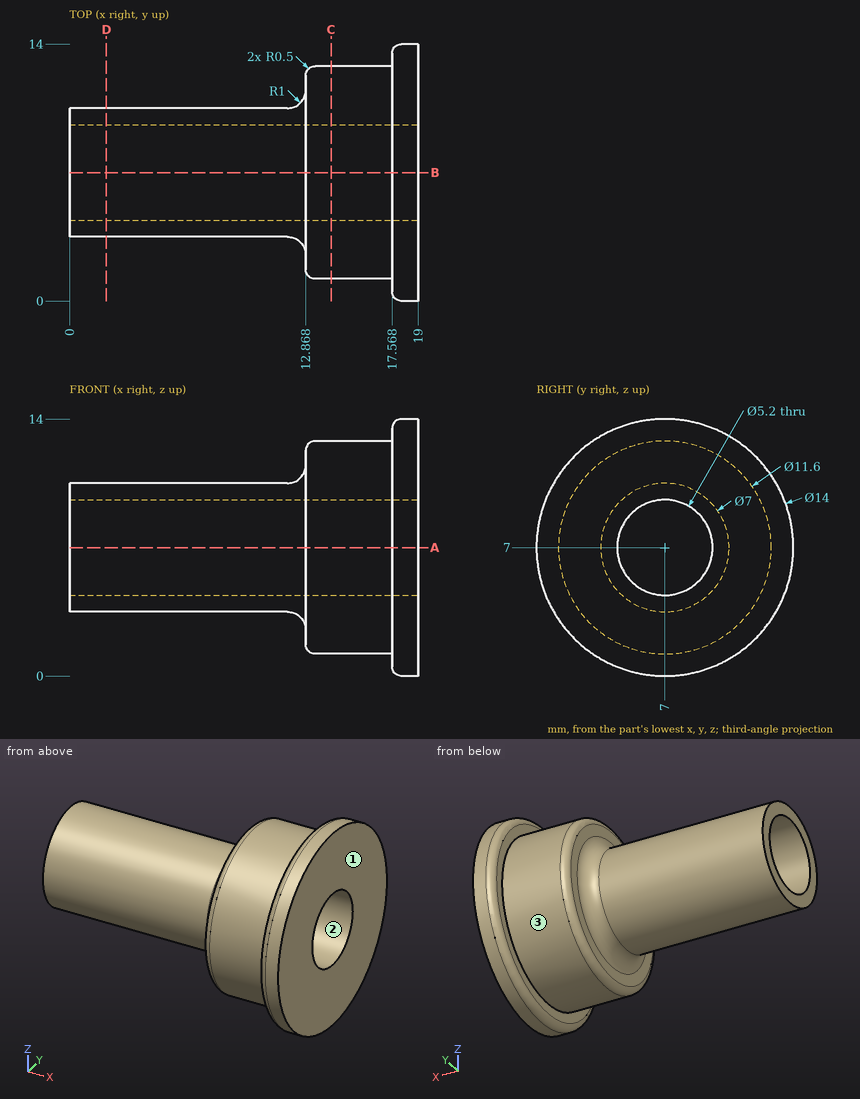
Drawing for the job (mm, zero at the part's lowest x, y, z). Round coordinates to 2 decimals unless told otherwise and drop trailing zeros. Write each loop counter-clockwise with the first axis right and the second up, starting at its lowest first coordinate (ties: lowest second). Pieces come first, ordered by that corner, then holes.
Item 1: Band-saw the part on D-D on x = 2. Write the cut outline in (y, z).
Filled in:
outline: circle Ø7 at (7, 7); hole circle Ø5.2 at (7, 7)
Item 2: Band-saw the part on A-A on z = 7. Write the cut outline in (x, y).
Filled in:
outline: (0, 3.5) - (11.87, 3.5) arc R1 cw to (12.87, 2.5) - (12.87, 1.7) arc R0.5 ccw to (13.37, 1.2) - (17.57, 1.2) - (17.57, 0.5) arc R0.5 ccw to (18.07, 0) - (19, 0) - (19, 4.4) - (0, 4.4) - close; (0, 9.6) - (19, 9.6) - (19, 14) - (18.07, 14) arc R0.5 ccw to (17.57, 13.5) - (17.57, 12.8) - (13.37, 12.8) arc R0.5 ccw to (12.87, 12.3) - (12.87, 11.5) arc R1 cw to (11.87, 10.5) - (0, 10.5) - close
Item 3: Drop flat-ended pins along their axis: pin 1 Ø3 at (x, y) = (16.5, 1.5) entering from -Z; pin 2 Ø1 at (x, y) = (13, 5) entering from +Z; pin 3 Ø2 at (x, y) = (13.5, 5.5) entering from +Z. Give the stop position or say it passes through.
Filled in:
pin 1: stops at z = 1.94
pin 2: stops at z = 12.57
pin 3: stops at z = 12.78
Item 4: Drill centre lines: L1, parallel to Z at x = 15.25, y = 7; L2, parallel to Z at x = 11.25, y = 7; L3, parallel to Y at x = 4, z = 6.25. Where is each one in solid material? Low to high.
Filled in:
L1: z = 1.2 to 4.4, 9.6 to 12.8
L2: z = 3.5 to 4.4, 9.6 to 10.5
L3: y = 3.58 to 4.51, 9.49 to 10.42
Item 5: Mould opens along Z. For the marked faces 1, 2 and 3 say: released by +Z, released by -Z, zero draft, split by the parting line, or undercut.
Filled in:
face 1: zero draft
face 2: undercut
face 3: split by the parting line
Item 6: Band-saw the part on C-C on x = 14.25. Write the cut outline in (y, z).
Filled in:
outline: circle Ø11.6 at (7, 7); hole circle Ø5.2 at (7, 7)
